Input: dimensioned drawing with shaded views. Units: mm. Origin: part minimum x, y, z. Give positions to 0.01 mm unless a question says otherwise; leave off trailing zeros. Loops run counter-clockwise (first coordinate to the right, second up) from the corner with the lowest first, then second, coordinate; pieces in that order, holes last.
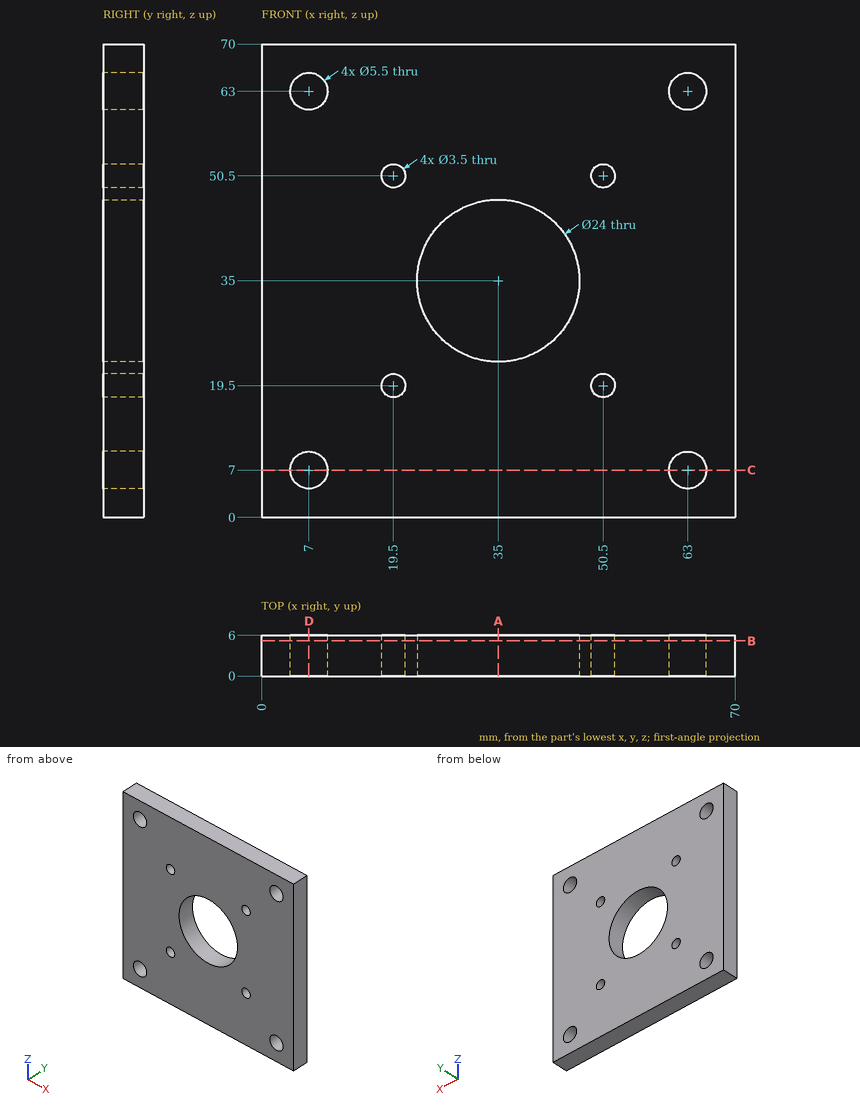
(1) First-contact query: pin 1 (5.5 mm diameter, centred on x = 19.5, z = 50.5, fed in from -Y); pin 2 (21.5 mm diameter, centred on x = 35, z = 35, fed in from -Y). Flat tips, straight axial feed; report the tip coordinate or a pass-through.
A:
pin 1: stops at y = 0
pin 2: passes through
(2) Section B-B, the plane y = 5.2. Count the separate pieces of the cut face and the enclosed holes in it, then the cut area to 3 significant figures.
A:
separate pieces: 1
enclosed holes: 9
area: 4,310 mm2
(3) Section A-A, the plane x = 35. Return the cut outline in (y, z).
A:
outline: (0, 0) - (6, 0) - (6, 23) - (0, 23) - close; (0, 47) - (6, 47) - (6, 70) - (0, 70) - close
(4) Section D-D, the plane x = 7. Return the cut outline in (y, z), then the cut area to 3 significant figures.
A:
outline: (0, 0) - (6, 0) - (6, 4.25) - (0, 4.25) - close; (0, 9.75) - (6, 9.75) - (6, 60.25) - (0, 60.25) - close; (0, 65.75) - (6, 65.75) - (6, 70) - (0, 70) - close
area: 354 mm2
(5) Ray query, line 1 along X through (y, z) = (1.4, 50.5); line 2 along X through (y, z) = (1.75, 7); line 3 along X through (y, z) = (1, 25.5). Return the intervals inside material, ascending.
A:
line 1: x = 0 to 17.75, 21.25 to 48.75, 52.25 to 70
line 2: x = 0 to 4.25, 9.75 to 60.25, 65.75 to 70
line 3: x = 0 to 27.67, 42.33 to 70
(6) Section C-C, the plane z = 7. Return the cut outline in (x, y).
A:
outline: (0, 0) - (4.25, 0) - (4.25, 6) - (0, 6) - close; (9.75, 0) - (60.25, 0) - (60.25, 6) - (9.75, 6) - close; (65.75, 0) - (70, 0) - (70, 6) - (65.75, 6) - close
